from build123d import *

# Parameters (mm, degrees)
SKETCH2_W                = 40
SKETCH2_H                = 40
BOSS_EXTRUDE1_DEPTH      = 20
BOSS_EXTRUDE1_DEPTH_BACK = 20
FILLET2_R                = 1
FILLET3_R                = 1
SKETCH3_W                = 37
SKETCH3_H                = 37
CUT_EXTRUDE1_DEPTH       = 0.5
CIRPATTERN1_COUNT        = 4
CIRPATTERN3_COUNT        = 2
CIRPATTERN3_ANGLE        = 90


with BuildPart() as part:
    # Sketch1 → Revolve1 (revolve)
    with BuildSketch(Plane.XY):
        with BuildLine():
            Line((0, 0), (180, 0))
            Line((180, 0), (180, 2))
            ThreePointArc((180, 2), (177.656854249, 7.656854249), (172, 10))
            Line((172, 10), (61.659544264, 10))
            Line((61.659544264, 10), (47.041451884, 10))
            Line((47.041451884, 10), (43, 3))
            Line((43, 3), (3, 3))
            Line((3, 3), (0, 0))
        make_face()
    revolve(axis=Axis((0, 0, 0), (1, 0, 0)))

    # Sketch2 → Boss-Extrude1 (add, two sides)
    with BuildSketch(Plane.XY) as boss_extrude1_sk:
        with Locations((172, 0)):
            Rectangle(SKETCH2_W, SKETCH2_H)
    extrude(amount=BOSS_EXTRUDE1_DEPTH)
    extrude(boss_extrude1_sk.sketch, amount=-BOSS_EXTRUDE1_DEPTH_BACK)

    # Fillet2
    fillet2_edges = [part.edges().sort_by_distance(p)[0] for p in [
        (152, -10, 0),
        (192, 20, 0),
        (192, 0, -20),
        (192, -20, 0),
        (172, -20, -20),
        (152, -20, 0),
        (152, 0, -20),
        (152, 20, 0),
        (172, 20, -20),
        (192, 0, 20),
        (172, 20, 20),
        (152, 0, 20),
        (172, -20, 20),
    ]]
    fillet(fillet2_edges, radius=FILLET2_R)

    # Fillet3
    fillet3_edges = [part.edges().sort_by_distance(p)[0] for p in [
        (3, -3, 0),
        (43, -3, 0),
        (47.041451884, -10, 0),
    ]]
    fillet(fillet3_edges, radius=FILLET3_R)

    # Sketch3 → Cut-Extrude1 (cut)
    with BuildSketch(Plane(origin=(0, 0, -20), x_dir=(-1, 0, 0), z_dir=(0, 0, -1))):
        with Locations((-172, 0)):
            Rectangle(SKETCH3_W, SKETCH3_H)
    cut_extrude1 = extrude(amount=-CUT_EXTRUDE1_DEPTH, mode=Mode.SUBTRACT)

    # CirPattern1: Cut-Extrude1 ×4 about axis
    cirpattern1_axis = Axis((0, 0, 0), (1, 0, 0))
    for i in range(1, CIRPATTERN1_COUNT):
        add(cut_extrude1.rotate(cirpattern1_axis, i * 360 / CIRPATTERN1_COUNT), mode=Mode.SUBTRACT)

    # CirPattern3: Cut-Extrude1 ×2 about axis
    cirpattern3_axis = Axis((172, 0, 0), (0, -1, 0))
    for i in range(1, CIRPATTERN3_COUNT):
        add(cut_extrude1.rotate(cirpattern3_axis, i * CIRPATTERN3_ANGLE / (CIRPATTERN3_COUNT - 1)), mode=Mode.SUBTRACT)


solid = part.part
The listing builds one solid part. Answer for the finished solid, in the listing's coordinates (mm). A direction names the side the tool comes from. Give positions to 0.01 mm unless a question says otherwise; leave off trailing zeros. Write each loop counter-clockwise with the first axis right and the second up, starting at its lowest first coordinate (ties: lowest second). Pieces come first, ordered by that corner, then holes. Notation, with made-up numbers: (-31, -40) - (-5, -40) arc R25 cw to (-5, -20) - close; hole circle Ø6 at (61.25, 30.25). An arc over 180 degrees is marked (long way). Use a Markdown table: item, result.
1. Section B-B on z = -15.5 is taken. Write down the section's boundary in (x, y).
Values follow:
| item | result |
|---|---|
| outline | (152, -19) arc R1 ccw to (153, -20) - (153.5, -20) - (153.5, -19.5) - (190.5, -19.5) - (190.5, -20) - (191, -20) arc R1 ccw to (192, -19) - (192, -18.5) - (191.5, -18.5) - (191.5, 18.5) - (192, 18.5) - (192, 19) arc R1 ccw to (191, 20) - (190.5, 20) - (190.5, 19.5) - (153.5, 19.5) - (153.5, 20) - (153, 20) arc R1 ccw to (152, 19) - close |
2. For a pull along X with two mould halves and no side action, classify faces 4 (the flat face through (191.5, 0, 0)), 5 (the flat face through (172, 0, 19.5)), 6 (the flat face through (172, -19.5, 0)), 7 (the cylindrical face through (22.65, -0.65, -2.93)) as released by +X, released by -X, zero draft, split by the parting line, or undercut.
Values follow:
| item | result |
|---|---|
| face 4 | released by +X |
| face 5 | undercut |
| face 6 | undercut |
| face 7 | zero draft |
3. Section A-A on x = 163.5 is taken. Write down the section's boundary in (y, z), plus the area to 3 significant figures.
Values follow:
| item | result |
|---|---|
| outline | (-20, -19) arc R1 ccw to (-19, -20) - (-18.5, -20) - (-18.5, -19.5) - (18.5, -19.5) - (18.5, -20) - (19, -20) arc R1 ccw to (20, -19) - (20, -18.5) - (19.5, -18.5) - (19.5, 18.5) - (20, 18.5) - (20, 19) arc R1 ccw to (19, 20) - (18.5, 20) - (18.5, 19.5) - (-18.5, 19.5) - (-18.5, 20) - (-19, 20) arc R1 ccw to (-20, 19) - (-20, 18.5) - (-19.5, 18.5) - (-19.5, -18.5) - (-20, -18.5) - close |
| area | 1,530 mm² |
4. Each of these flat-tipped pins is pushed along its axis until it touches: P1, Ø0.6, axis at x = 192, y = 2.5, coming from the +Z side; P2, Ø0.6, axis at x = 174.5, z = 19.5, coming from the +Y side; P3, Ø2, axis at x = 172.5, z = 1, coming from the -Y side. Where does it stop, or does it pass through?
Values follow:
| item | result |
|---|---|
| P1 | stops at z = 19.71 |
| P2 | stops at y = 19.98 |
| P3 | stops at y = -19.5 |
5. Find the intervals of material crossed by probe 1 along X at (y, z) = (9, -9); probe 2 along Z at (x, y) = (165, -2.5); probe 3 along Z at (x, y) = (125.5, 0), in increasing order. Write a range as from..to.
Values follow:
| item | result |
|---|---|
| probe 1 | x = 152..191.5 |
| probe 2 | z = -19.5..19.5 |
| probe 3 | z = -10..10 |
6. A tool of negligible diameter and unlimited length cuts with its end or side. For faces 1 (the flat face through (152, -9, 9)), 2 (the flat face through (172, 19.5, 0)), 3 (the flat face through (172, 0, -19.5)), from which of +Z, -Z, +X, -X, +Y, -Y can it reach the whole face along a straight path? Write none if from no direction.
Values follow:
| item | result |
|---|---|
| face 1 | -X |
| face 2 | +Y |
| face 3 | -Z |
7. Section D-D on x = 50 is taken. Write down the section's boundary in (y, z), plus the area to 3 significant figures.
Values follow:
| item | result |
|---|---|
| outline | circle Ø20 at (0, 0) |
| area | 314 mm² |
